Could you check a few things on this model? Use its own coordinates, in mm. A direction names the side the tool comes from. Give positions to 0.01 mm unless a question says otherwise; leave off trailing zeros. Loops run counter-clockwise (first coordinate to the right, second up) from the corner with the lowest first, then second, coordinate; pieces in that order, holes last. Notation, with made-up numbers: (17, -17) - (58, -17) arc R20 ccw to (58, 1) - close; hole circle Ø9 at (65, -29). An arc over 180 degrees is marked (long way). Write each question's results on one line, items separated by ' | '. Start each with the question number.
(1) Suppose I cut it at A-A (y = 0). Please give me the cut outline in (x, z).
(2) For pin 1 (6 mm diameter, centred on x = 112, z = -14, fed in from +Y); pin 2 (2 mm diameter, centred on x = -134.5, z = 2, fed in from +Y); pin 3 (10 mm diameter, centred on x = 122, z = -1.5, fed in from +Y), each with a flat end and sliding along its axis, tell me the tip position at first contact or that it passes through.
(3) On a 3-axis mill with a long thin cutter (end or side, diameter ignored), from which of +Z, -Z, +X, -X, +Y, -Y can I reach the whole of each face in a straight line? I mean faces 1 (the face through (-52.569, -236.733, -2.822)), 2 (the face through (-84, 229, 20.5)). Say none if no direction works.
(4) I need wall thicknesses on line 1 (Y direction, x = 148, z = -4); line 2 (X direction, y = -4, z = 15); line 3 (X direction, y = 250, z = -21.5). Which ranges of each line are inside material? Lowest first, please.
(5) Suppose I cut it at C-C (z = -11). Count the separate pieces of the cut face and the enclosed holes in it, and give its area (3 significant figures).
(6) If we mould it in two halves opening along X, with no side actions, what happens to faces 3 (the face through (267.16, -100.75, 0.36)), 4 (the face through (-119, 213, -25.5)), 5 (the face through (-41.397, 315.294, 0.357))? For each: released by +X, released by -X, zero draft, split by the parting line, or undercut.
(7) Suppose I cut it at B-B (x = -51.5). Please give me the cut outline in (y, z), and give its area (3 significant figures).
from build123d import *

# Parameters (mm, degrees)
SKETCH1_R           = 318
SKETCH1_R_2         = 242.5
BOSS_EXTRUDE1_DEPTH = 25.5
SKETCH2_R           = 279
CUT_EXTRUDE1_DEPTH  = 5
SKETCH3_R           = 11
CUT_EXTRUDE2_DEPTH  = 27.5


with BuildPart() as part:
    # Sketch1 → Boss-Extrude1 (new body, symmetric)
    with BuildSketch(Plane.XY):
        Circle(SKETCH1_R)
        Circle(SKETCH1_R_2, mode=Mode.SUBTRACT)
    extrude(amount=BOSS_EXTRUDE1_DEPTH, both=True)

    # Sketch2 → Cut-Extrude1 (cut)
    with BuildSketch(Plane.XY.offset(25.5)):
        Circle(SKETCH2_R)
    extrude(amount=-CUT_EXTRUDE1_DEPTH, mode=Mode.SUBTRACT)

    # Sketch3 → Cut-Extrude2 (cut, symmetric)
    with BuildSketch(Plane.XY):
        with Locations((0, 296)):
            Circle(SKETCH3_R)
        with Locations((51.399860589, 291.503094892)):
            Circle(SKETCH3_R)
        with Locations((101.237962424, 278.149015753)):
            Circle(SKETCH3_R)
        with Locations((148, 256.34351952)):
            Circle(SKETCH3_R)
        with Locations((190.265132467, 226.749155163)):
            Circle(SKETCH3_R)
        with Locations((226.749155163, 190.265132467)):
            Circle(SKETCH3_R)
        with Locations((256.34351952, 148)):
            Circle(SKETCH3_R)
        with Locations((278.149015753, 101.237962424)):
            Circle(SKETCH3_R)
        with Locations((291.503094892, 51.399860589)):
            Circle(SKETCH3_R)
        with Locations((296, 0)):
            Circle(SKETCH3_R)
        with Locations((291.503094892, -51.399860589)):
            Circle(SKETCH3_R)
        with Locations((278.149015753, -101.237962424)):
            Circle(SKETCH3_R)
        with Locations((256.34351952, -148)):
            Circle(SKETCH3_R)
        with Locations((226.749155163, -190.265132467)):
            Circle(SKETCH3_R)
        with Locations((190.265132467, -226.749155163)):
            Circle(SKETCH3_R)
        with Locations((148, -256.34351952)):
            Circle(SKETCH3_R)
        with Locations((101.237962424, -278.149015753)):
            Circle(SKETCH3_R)
        with Locations((51.399860589, -291.503094892)):
            Circle(SKETCH3_R)
        with Locations((0, -296)):
            Circle(SKETCH3_R)
        with Locations((-51.399860589, -291.503094892)):
            Circle(SKETCH3_R)
        with Locations((-101.237962424, -278.149015753)):
            Circle(SKETCH3_R)
        with Locations((-148, -256.34351952)):
            Circle(SKETCH3_R)
        with Locations((-190.265132467, -226.749155163)):
            Circle(SKETCH3_R)
        with Locations((-226.749155163, -190.265132467)):
            Circle(SKETCH3_R)
        with Locations((-256.34351952, -148)):
            Circle(SKETCH3_R)
        with Locations((-278.149015753, -101.237962424)):
            Circle(SKETCH3_R)
        with Locations((-291.503094892, -51.399860589)):
            Circle(SKETCH3_R)
        with Locations((-296, 0)):
            Circle(SKETCH3_R)
        with Locations((-291.503094892, 51.399860589)):
            Circle(SKETCH3_R)
        with Locations((-278.149015753, 101.237962424)):
            Circle(SKETCH3_R)
        with Locations((-256.34351952, 148)):
            Circle(SKETCH3_R)
        with Locations((-226.749155163, 190.265132467)):
            Circle(SKETCH3_R)
        with Locations((-190.265132467, 226.749155163)):
            Circle(SKETCH3_R)
        with Locations((-148, 256.34351952)):
            Circle(SKETCH3_R)
        with Locations((-101.237962424, 278.149015753)):
            Circle(SKETCH3_R)
        with Locations((-51.399860589, 291.503094892)):
            Circle(SKETCH3_R)
    extrude(amount=CUT_EXTRUDE2_DEPTH, both=True, mode=Mode.SUBTRACT)


solid = part.part
Output values:
1) outline: (-318, -25.5) - (-307, -25.5) - (-307, 25.5) - (-318, 25.5) - close; (-285, -25.5) - (-242.5, -25.5) - (-242.5, 20.5) - (-279, 20.5) - (-279, 25.5) - (-285, 25.5) - close; (242.5, -25.5) - (285, -25.5) - (285, 25.5) - (279, 25.5) - (279, 20.5) - (242.5, 20.5) - close; (307, -25.5) - (318, -25.5) - (318, 25.5) - (307, 25.5) - close
2) pin 1: y = 298.74 | pin 2: y = 288.62 | pin 3: y = 295.69
3) face 1: +Z, -Z | face 2: +Z
4) line 1: -281.46 to -267.34, -245.34 to -192.1, 192.1 to 245.34, 267.34 to 281.46 | line 2: -317.97 to -306.25, -285.75 to -242.47, 242.47 to 285.75, 306.25 to 317.97 | line 3: -196.53 to -156.99, -139.01 to 139.01, 156.99 to 196.53
5) separate pieces: 1 | enclosed holes: 37 | area: 119,000 mm2
6) face 3: undercut | face 4: zero draft | face 5: split by the parting line
7) outline: (-313.8, -25.5) - (-302.5, -25.5) - (-302.5, 25.5) - (-313.8, 25.5) - close; (-280.5, -25.5) - (-236.97, -25.5) - (-236.97, 20.5) - (-274.21, 20.5) - (-274.21, 25.5) - (-280.5, 25.5) - close; (236.97, -25.5) - (280.5, -25.5) - (280.5, 25.5) - (274.21, 25.5) - (274.21, 20.5) - (236.97, 20.5) - close; (302.5, -25.5) - (313.8, -25.5) - (313.8, 25.5) - (302.5, 25.5) - close | area: 5,220 mm2
